CAD build for the part. Positions are in the model's coordinates, mm. Face numbers are marked on the shaded views. Round coordinates to 2 decimals unless told otherwise and drop trailing zeros. Loops run counter-clockwise (first coordinate to the right, second up) from the corner with the lowest first, then second, coordinate; pieces in that order, holes last. Notation, with made-up numbers: (54, -22.5) -> (64, -22.5) arc R10 cw to (64, -12.5) -> close; hole circle Ø6 at (47.25, 44). An arc over 180 degrees is marked (long way). Answer as CSV lines item,"result".
```python
from build123d import *

# Parameters (mm, degrees)
SKETCH1_R           = 35
SKETCH1_R_2         = 30
BOSS_EXTRUDE1_DEPTH = 18
SKETCH2_R           = 3
BOSS_EXTRUDE2_DEPTH = 10
SKETCH3_R           = 1.75
CUT_EXTRUDE1_DEPTH  = 53.668776329


with BuildPart() as part:
    # Sketch1 → Boss-Extrude1 (new body)
    with BuildSketch(Plane(origin=(0, 0, 0), x_dir=(1, 0, 0), z_dir=(0, 1, 0))):
        with Locations(Location((0, 0, 0), (0, 0, 270))):
            Circle(SKETCH1_R)
        with Locations(Location((0, 0, 0), (0, 0, 270))):
            Circle(SKETCH1_R_2, mode=Mode.SUBTRACT)
    extrude(amount=BOSS_EXTRUDE1_DEPTH)

    # Sketch2 → Boss-Extrude2 (add)
    with BuildSketch(Plane(origin=(0, 0, 0), x_dir=(1, 0, 0), z_dir=(0, 1, 0))):
        with Locations((0, 29)):
            Circle(SKETCH2_R)
        with Locations((15.678583706, 24.396352452)):
            Circle(SKETCH2_R)
        with Locations((26.379327865, 12.047035377)):
            Circle(SKETCH2_R)
        with Locations((28.704821815, -4.12713031)):
            Circle(SKETCH2_R)
        with Locations((21.916737656, -18.990961284)):
            Circle(SKETCH2_R)
        with Locations((8.170244148, -27.825296235)):
            Circle(SKETCH2_R)
        with Locations((-8.170244148, -27.825296235)):
            Circle(SKETCH2_R)
        with Locations((-21.916737656, -18.990961284)):
            Circle(SKETCH2_R)
        with Locations((-28.704821815, -4.12713031)):
            Circle(SKETCH2_R)
        with Locations((-26.379327865, 12.047035377)):
            Circle(SKETCH2_R)
        with Locations((-15.678583706, 24.396352452)):
            Circle(SKETCH2_R)
    extrude(amount=BOSS_EXTRUDE2_DEPTH)

    # Sketch3 → Cut-Extrude1 (cut, through all)
    with BuildSketch(Plane(origin=(0, 18, 0), x_dir=(1, 0, 0), z_dir=(0, 1, 0))):
        with Locations(Location((0, 32.5, 0), (0, 0, 270))):
            Circle(SKETCH3_R)
        with Locations(Location((32.5, 0, 0), (0, 0, 270))):
            Circle(SKETCH3_R)
        with Locations(Location((0, -32.5, 0), (0, 0, 270))):
            Circle(SKETCH3_R)
        with Locations(Location((-32.5, 0, 0), (0, 0, 270))):
            Circle(SKETCH3_R)
    extrude(amount=-CUT_EXTRUDE1_DEPTH, mode=Mode.SUBTRACT)


solid = part.part
```
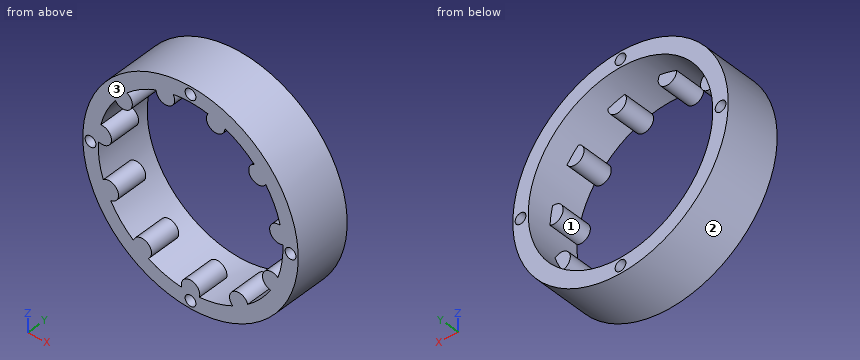
Q1. Two-plate mould, pull along X, no slides. Class the marked faces 1, 2 and 3: pulls with the +X half, pulls with the -X half, needs draft (parallel to the pull), parting line crosses it, or undercut.
Results:
face 1,"undercut"
face 2,"parting line crosses it"
face 3,"needs draft"
Q2. Slice it at C-C, the plane y = 14. Give the cut face in (x, z), and give its area (3 significant figures).
Results:
outline,"circle Ø70 at (0, 0); hole circle Ø3.5 at (-32.5, 0); hole circle Ø60 at (0, 0); hole circle Ø3.5 at (0, -32.5); hole circle Ø3.5 at (0, 32.5); hole circle Ø3.5 at (32.5, 0)"
area,"983 mm2"
Q3. Slice it at B-B, the plane z = 0. Give the cut face in (x, y).
Results:
outline,"(-35, 0) -> (-34.25, 0) -> (-34.25, 18) -> (-35, 18) -> close; (-30.75, 0) -> (-30, 0) -> (-30, 18) -> (-30.75, 18) -> close; (30, 0) -> (30.75, 0) -> (30.75, 18) -> (30, 18) -> close; (34.25, 0) -> (35, 0) -> (35, 18) -> (34.25, 18) -> close"
Q4. Slice it at A-A, the plane x = 0. Give the cut face in (y, z).
Results:
outline,"(0, -35) -> (18, -35) -> (18, -34.25) -> (0, -34.25) -> close; (0, -30.75) -> (18, -30.75) -> (18, -30) -> (10, -30) -> (10, -26) -> (0, -26) -> close; (0, 30) -> (18, 30) -> (18, 30.75) -> (0, 30.75) -> close; (0, 34.25) -> (18, 34.25) -> (18, 35) -> (0, 35) -> close"
Q5. Drop flat-ended pins along their axis: pin 1 Ø3.5 at (x, z) = (-27.5, 5.5) entering from +Y; pin 2 Ø4 at (x, y) = (9, 12.5) entering from +Z; pin 3 Ø6 at (x, y) = (-19, 15) entering from +Z. Give the stop position or say it passes through.
Results:
pin 1,"y = 10"
pin 2,"z = 34.29"
pin 3,"z = 31.13"
Q6. Slice it at D-D, the plane x = -17. Give the cut face in (y, z), and give its area (3 significant figures).
Results:
outline,"(0, -30.59) -> (18, -30.59) -> (18, -24.72) -> (10, -24.72) -> (10, -21.7) -> (0, -21.7) -> close; (0, 24.72) -> (18, 24.72) -> (18, 30.59) -> (0, 30.59) -> close"
area,"242 mm2"
Q7. Probe L1, parallel to X at y = 12, z = 0; L2, parallel to X at y = 7.75, z = -8; L3, parallel to Z at x = 27, y = 2.5. List the from-to ranges inside material, lowest first. Write a range as [from, to].
Results:
L1,"[-35, -34.25], [-30.75, -30], [30, 30.75], [34.25, 35]"
L2,"[-34.07, -28.91], [28.91, 34.07]"
L3,"[-22.27, -9.11], [1.66, 6.6], [13.08, 22.27]"
